Here's the drawing with two shaded views (mm, measured from the low corner). I have some questions. Coordinates: 2 decimals unless noted, no trailing zeros. Write each loop counter-clockwise with the first axis right and the second up, starting at its lowest first coordinate (ties: lowest second). Pieces come first, ordered by that corner, then holes.
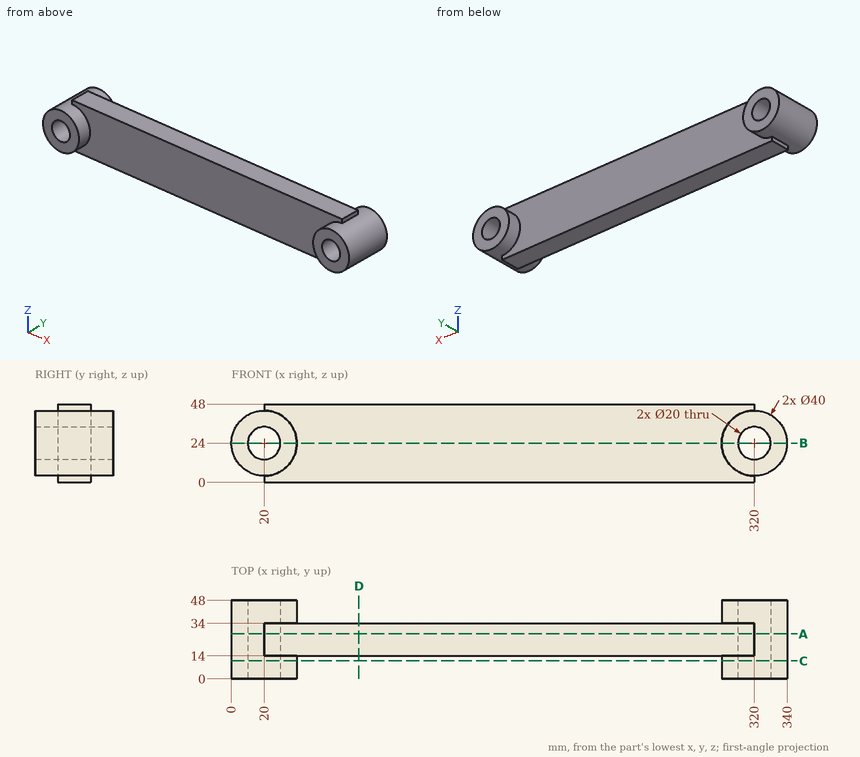
1. I want a section at A-A on y = 27.5. Please give me the cut outline in (x, z), plus the area to 3 significant figures.
Verdict:
outline: (20, 0) - (320, 0) - (320, 4) arc R20 ccw to (320, 44) - (320, 48) - (20, 48) - (20, 44) arc R20 ccw to (20, 4) - close; hole circle Ø20 at (20, 24); hole circle Ø20 at (320, 24)
area: 15,000 mm2
2. I want a section at B-B on z = 24. Please give me the cut outline in (x, y).
Verdict:
outline: (0, 0) - (10, 0) - (10, 48) - (0, 48) - close; (30, 0) - (40, 0) - (40, 14) - (300, 14) - (300, 0) - (310, 0) - (310, 48) - (300, 48) - (300, 34) - (40, 34) - (40, 48) - (30, 48) - close; (330, 0) - (340, 0) - (340, 48) - (330, 48) - close
3. I want a section at C-C on y = 11. Please give me the cut outline in (x, z), plus the area to 3 significant figures.
Verdict:
outline: circle Ø40 at (20, 24); circle Ø40 at (320, 24); hole circle Ø20 at (20, 24); hole circle Ø20 at (320, 24)
area: 1,880 mm2
4. Please list where these lines run through material, in increasing order: line 1 along X through (y, z) = (27, 24); line 2 along X through (y, z) = (13, 24); line 3 along X through (y, z) = (44, 30.5).
Verdict:
line 1: x = 0 to 10, 30 to 310, 330 to 340
line 2: x = 0 to 10, 30 to 40, 300 to 310, 330 to 340
line 3: x = 1.09 to 12.4, 27.6 to 38.91, 301.09 to 312.4, 327.6 to 338.91
5. I want a section at D-D on x = 78. Please give me the cut outline in (y, z), plus the area to 3 significant figures.
Verdict:
outline: (14, 0) - (34, 0) - (34, 48) - (14, 48) - close
area: 960 mm2
6. For pin 1 (3 mm diameter, centred on y = 21.5, z = 2, fed in from -X); pin 2 (1 mm diameter, centred on y = 27, z = 24.5, fed in from +X); pin 3 (8 mm diameter, centred on y = 38, z = 34, fed in from +X), each with a flat end and sliding along its axis, tell me the tip position at first contact or that it passes through.
Verdict:
pin 1: stops at x = 20
pin 2: stops at x = 340
pin 3: stops at x = 339.08
